Input: part model. Units: mm. Frame: model coordinates. Coordinates: 2 decimals unless noted, no trailing zeros. Write each loop counter-clockwise with the first axis right and the second up, starting at its lowest first coordinate (ties: lowest second). Pieces come first, ordered by that corner, then holes. Notation, with made-up numbers: M -35.75,73 L 0.25,73 A29 cw 0.25,108 Z; hole C 59.5,13 d8. An arc over 180 degrees is marked long. Write each question's results on one line, items separated by ' | '. Start each with the question number.
1. Section query B-B, the plane x = -65. Output: boundary loops of the cut face in (y, z).
2. Section query A-A, the plane y = 15.5. Output: boundary loops of the cut face in (x, z).
3. Section query C-C, the plane z = -114. Output: boundary loops of the cut face in (x, y).
4. First-contact query: pin 1 (4 mm diameter, centred on y = 10.5, z = -42, fed in from +X); pin 2 (6 mm diameter, centred on x = -143, z = -57.5, fed in from +Y); pin 3 (3 mm diameter, centred on y = 10, z = -42, fed in from -X). Flat tips, straight axial feed; report the tip coordinate or a pass-through.
5. Ray query, probe 1 along Z at (x, y) = (-1.3, 10); probe 2 along Z at (x, y) = (-1, 30); probe 3 along Y at (x, z) = (-0.7, -98.58). Return the intervals inside material, ascending.
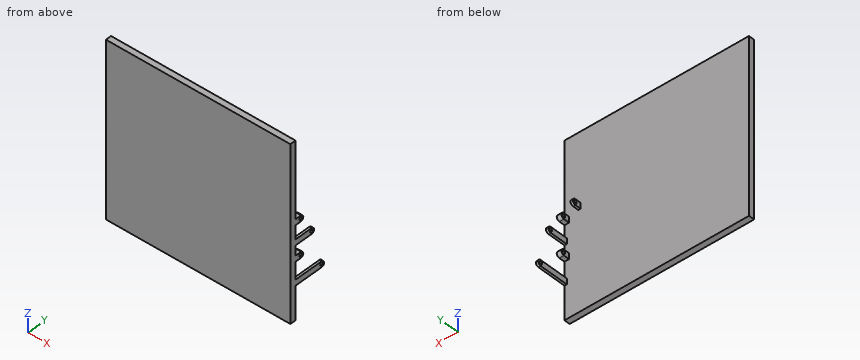
Autodesk Inventor part; units mm, degrees
ref_plane "工作平面1" through (-12, 0, -130) normal (1, 0, 0) x (0, 0, -1)
ref_plane "YZ Plane" through (0, 0, 0) normal (1, 0, 0) x (0, 1, 0)
ref_plane "XZ Plane" through (0, 0, 0) normal (0, 1, 0) x (-1, 0, 0)
sketch "草圖1" plane through (0, 0, 0) normal (0, 1, 0) x (-1, 0, 0)
  line L0 (0, 0) -> (160, 0)
  line L1 (160, 0) -> (160, -130)
  line L2 (160, -130) -> (0, -130)
  line L3 (0, -130) -> (0, 0)
  dimension "d0" = 160
  dimension "d1" = 130
extrude "擠出1" add sketch "草圖1" along normal blind 5
sketch "草圖2" plane through (0, 0, 0) normal (1, 0, 0) x (0, 0, -1)
  line L0 (130, 0) -> (0, 0)
  line L1 (65, 0) -> (65, 20.4)
  line L2 (65, 20.4) -> (65, 0) construction
  line L3 (62.5, 20.4) -> (62.5, 0)
  line L4 (67.5, 0) -> (67.5, 20.4)
  arc A0 (67.5, 20.4) -> (62.5, 20.4) centre (65, 20.4) ccw
  arc A1 (62.5, 0) -> (67.5, 0) centre (65, 0) ccw construction
  line L5 (67.5, 0) -> (62.5, 0)
  circle A2 centre (65, 20.4) radius 1.25
  point P0 (65, 10.2)
  dimension "d4" = 20.4
  dimension "d5" = 5
  dimension "d6" = 2.5
extrude "擠出2" add sketch "草圖2" against normal blind 2
sketch "草圖3" plane through (0, 0, 0) normal (1, 0, 0) x (0, 0, -1)
  line L0 (130, 0) -> (0, 0) construction
  arc A0 (67.5, 20.4) -> (62.5, 20.4) centre (65, 20.4) ccw
  line L1 (65, 20.4) -> (48.2, 20.4) construction
  line L2 (48.2, 20.4) -> (48.2, 10) construction
  line L3 (48.2, 10) -> (48.2, 0) construction
  line L4 (45.7, 10) -> (45.7, 0)
  line L5 (50.7, 0) -> (50.7, 10)
  arc A1 (50.7, 10) -> (45.7, 10) centre (48.2, 10) ccw
  arc A2 (45.7, 0) -> (50.7, 0) centre (48.2, 0) ccw construction
  circle A3 centre (48.2, 10) radius 1.25
  line L6 (50.7, 0) -> (45.7, 0)
  line L7 (65, 20.4) -> (42, 20.4) construction
  line L8 (42, 20.4) -> (42, 10) construction
  line L9 (42, 10) -> (42, 0) construction
  line L10 (39.5, 10) -> (39.5, 0)
  line L11 (44.5, 0) -> (44.5, 10)
  arc A4 (44.5, 10) -> (39.5, 10) centre (42, 10) ccw
  arc A5 (39.5, 0) -> (44.5, 0) centre (42, 0) ccw construction
  circle A6 centre (42, 10) radius 1.25
  line L12 (44.5, 0) -> (39.5, 0)
  circle A7 centre (65, 20.4) radius 1.25
  line L13 (65, 20.4) -> (78.6, 20.4) construction
  line L14 (78.6, 20.4) -> (78.6, 10) construction
  line L15 (78.6, 10) -> (78.6, 0) construction
  line L16 (76.1, 10) -> (76.1, 0)
  line L17 (81.1, 0) -> (81.1, 10)
  arc A8 (81.1, 10) -> (76.1, 10) centre (78.6, 10) ccw
  arc A9 (76.1, 0) -> (81.1, 0) centre (78.6, 0) ccw construction
  circle A10 centre (78.6, 10) radius 1.25
  line L18 (81.1, 0) -> (76.1, 0)
  line L19 (81.1, 0) -> (76.1, 0)
  line L20 (0, 0) -> (130, 0)
  line L21 (65, 20.4) -> (65, 30.17) construction
  line L22 (65, 30.17) -> (98.58, 30.17) construction
  line L23 (98.58, 30.17) -> (98.58, 0) construction
  line L24 (96.08, 30.17) -> (96.08, 0)
  line L25 (101.08, 0) -> (101.08, 30.17)
  arc A11 (101.08, 30.17) -> (96.08, 30.17) centre (98.58, 30.17) ccw
  arc A12 (96.08, 0) -> (101.08, 0) centre (98.58, 0) ccw construction
  circle A13 centre (98.58, 30.17) radius 1.25
  line L26 (101.08, 0) -> (96.08, 0)
  point P0 (48.2, 5)
  point P1 (42, 5)
  point P2 (78.6, 5)
  point P3 (98.58, 15.085)
  dimension "d9" = 16.8
  dimension "d11" = 10.4
  dimension "d12" = 5
  dimension "d13" = 2.5
  dimension "d14" = 23
  dimension "d15" = 10.4
  dimension "d16" = 5
  dimension "d17" = 2.5
  dimension "d20" = 13.6
  dimension "d21" = 10.4
  dimension "d22" = 5
  dimension "d23" = 2.5
  dimension "d24" = 9.77
  dimension "d25" = 33.58
  dimension "d26" = 5
  dimension "d27" = 2.5
extrude "擠出3" add sketch "草圖3" against normal blind 2 contours A1 L5 L6 L4 | L24 A11 L25 L20 | L16 A8 L17 L18 | L12 L10 A4 L11
sketch "草圖4" plane through (-160, 0, 0) normal (0, 0, 1) x (1, 0, 0)
  line L0 (160, 0) -> (0, 0)
  line L1 (160, 0) -> (160, 5)
  line L2 (0, 5) -> (160, 5)
  line L3 (0, 0) -> (0, 5)
extrude "擠出4" add sketch "草圖4" along normal blind 20
sketch "草圖5" plane through (-2, 0, 0) normal (-1, 0, 0) x (0, 0, 1)
  line L0 (-45.7, 5) -> (-50.7, 5)
  line L1 (-45.7, 5) -> (-45.7, 10)
  arc A0 (-45.7, 10) -> (-50.7, 10) centre (-48.2, 10) ccw
  line L2 (-50.7, 10) -> (-50.7, 5)
  circle A1 centre (-48.2, 10) radius 1.25
  line L3 (-76.1, 5) -> (-81.1, 5)
  line L4 (-76.1, 5) -> (-76.1, 10)
  arc A2 (-76.1, 10) -> (-81.1, 10) centre (-78.6, 10) ccw
  line L5 (-81.1, 10) -> (-81.1, 5)
  circle A3 centre (-78.6, 10) radius 1.25
  point P0 (0, 0)
extrude "擠出5" add sketch "草圖5" along normal blind 2
ref_plane "工作平面1" through (-12, 0, -130) normal (1, 0, 0) x (0, 0, -1)
sketch "草圖6" plane through (-12, 0, -130) normal (1, 0, 0) x (0, 0, -1)
  line L0 (-90.5, 5) -> (-85.5, 5)
  line L1 (-90.5, 5) -> (-90.5, 10)
  arc A0 (-85.5, 10) -> (-90.5, 10) centre (-88, 10) ccw
  line L2 (-85.5, 10) -> (-85.5, 5)
  circle A1 centre (-88, 10) radius 1.25
  point P0 (-130, 0)
extrude "擠出6" add sketch "草圖6" against normal blind 2
extrude "擠出7" cut sketch "草圖6" along normal blind 20
Answer:
1) outline: M 0,-130 L 5,-130 L 5,20 L 0,20 Z
2) outline: M -2,-101.08 L 0,-101.08 L 0,-96.08 L -2,-96.08 Z; M -2,-67.5 L 0,-67.5 L 0,-62.5 L -2,-62.5 Z
3) outline: M -160,0 L 0,0 L 0,5 L -160,5 Z
4) pin 1: x = -12 | pin 2: y = 5 | pin 3: x = -14
5) probe 1: -101.08 to -96.08, -81.1 to -79.85, -77.35 to -76.1, -67.5 to -62.5, -50.7 to -49.45, -46.95 to -45.7 | probe 2: -101.08 to -99.82, -97.34 to -96.08 | probe 3: 0 to 28.92, 31.42 to 32.67
